Build history of the part. All positions in model axes, mm. A direction names the side the tool comes from. Round coordinates to 2 decimals unless told otherwise and drop trailing zeros. Order: outer loops, then holes, each group sorted by start corner. A loop starts at its lowest first (then second) coordinate and runs counter-clockwise, first axis right, second up. Notation, with made-up numbers: (1, 29) -> (22, 29) arc R13 ccw to (22, 51) -> close; hole circle Ø4 at (15.5, -1). An arc over 180 degrees is marked (long way). Use a Markdown table: item, result. Add a question column.
Item 1: Two-plate mould, pull along Y, no slides. Class faces 1 (the face through (4.59, 2.68, 16.08)), 2 (the face through (-6.2, 2, 11.486)), 3 (the face through (-1.38, 6.2, 2.09)): released by +Y, released by -Y, zero draft, split by the parting line, or undercut.
Item 2: Pin check, flat tips, straight feed: pin 1 (3 mm diameter, centred on y = 6, z = 1.5, fed in from +X); pin 2 (5 mm diameter, centred on y = 2.5, z = -1, fed in from -X); pin 3 (4 mm diameter, centred on x = -3.5, z = 11, fed in from +Y). Stop position of each tip, or through.
Item 3: 3-axis set-ups, long thin cutter, end or side, ignore diameter. For faces 4 (the face through (-4.59, -2.68, 16.08)), 5 (the face through (0, 0, -7.564)): which of +Z, -Z, +X, -X, +Y, -Y reach the whole face in a straight line?
Item 4: Probe L1, parallel to Z at x = -1.5, y = -5; L2, parallel to X at y = -3.25, z = 16; L3, parallel to Y at x = 0.5, z = 14.75. List the from-to ranges inside material, lowest first.
Item 5: Slice it at A-A, the plane z = 6. Give the cut face in (x, y), plus the area to 3 significant figures.
from build123d import *

# Parameters (mm, degrees)
F3_DEPTH = 3.175


# Not quite as in the source:
# - a fillet or chamfer that OpenCascade refuses, or shapes differently, is made with other operations: its cross-section is extruded or revolved along the edge and cut away or added


with BuildPart() as f1:
    # F0 (on Front) → F1 (revolve)
    with BuildSketch(Plane.XZ):
        Polygon((9.525, 17.8360301112), (0, 17.8360301112), (0, -7.5639698888), (6.35, -7.5639698888), (6.35, 11.4860301112), (9.525, 11.4860301112), align=None)
    revolve(axis=Axis((0, 0, 2.9950272292), (0, 0, -1)))

    # F2 (on face) → F3 (cut)
    with BuildSketch(Plane.XY.offset(17.8360301112)):
        Polygon((-3.001152127, -5.3557559125), (3.1376446132, -5.2769519389), (6.1387967402, 0.0788039736), (3.001152127, 5.3557559125), (-3.1376446132, 5.2769519389), (-6.1387967402, -0.0788039736), align=None)
    extrude(amount=-F3_DEPTH, mode=Mode.SUBTRACT)

    # F4: fillet of radius 6.35 on 1 edges, made by hand

    # F4_s1 → F4_t2 (revolve, cut)
    with BuildSketch(Plane.XZ):
        with BuildLine():
            ThreePointArc((3.175, 17.8360301112), (7.6651280605, 15.9761581718), (9.525, 11.4860301112))
            Line((9.525, 11.4860301112), (9.525, 17.8360301112))
            Line((9.525, 17.8360301112), (3.175, 17.8360301112))
        make_face()
    revolve(axis=Axis((0, 0, 17.8360301112), (0, 0, -1)), mode=Mode.SUBTRACT)


solid = f1.part
Check sheet entries:
| question | item | result |
|---|---|---|
| 1 | face 1 | undercut |
| 1 | face 2 | zero draft |
| 1 | face 3 | split by the parting line |
| 2 | pin 1 | x = 4.48 |
| 2 | pin 2 | x = -6.35 |
| 2 | pin 3 | y = 9.4 |
| 3 | face 4 | +Z |
| 3 | face 5 | -Z, +X, -X, +Y, -Y |
| 4 | L1 | -7.56 to 14.66 |
| 4 | L2 | -6.92 to -4.25, 4.27 to 6.92 |
| 4 | L3 | -8.61 to -5.31, 5.32 to 8.61 |
| 5 | outline | circle Ø12.7 at (0, 0) |
| 5 | area | 127 mm2 |
